The figure shows three views and two pictorial views of one solid part (mm, origin at its lowest corner). Answer the questions. A direction names the side the tool comes from. Coordinates: 2 decimals unless noted, no trailing zeros. Loops run counter-clockwise (first coordinate to the right, second up) from the corner with the lowest first, then second, coordinate; pieces in that order, holes last. Notation, with made-up numbers: (64.25, 77.5) -> (104.25, 77.5) arc R31 ccw to (104.25, 111.5) -> close; hole circle Ø1 at (-27.75, -4). An arc over 180 degrees is marked (long way). Use a Markdown table: item, result. Add a question column.
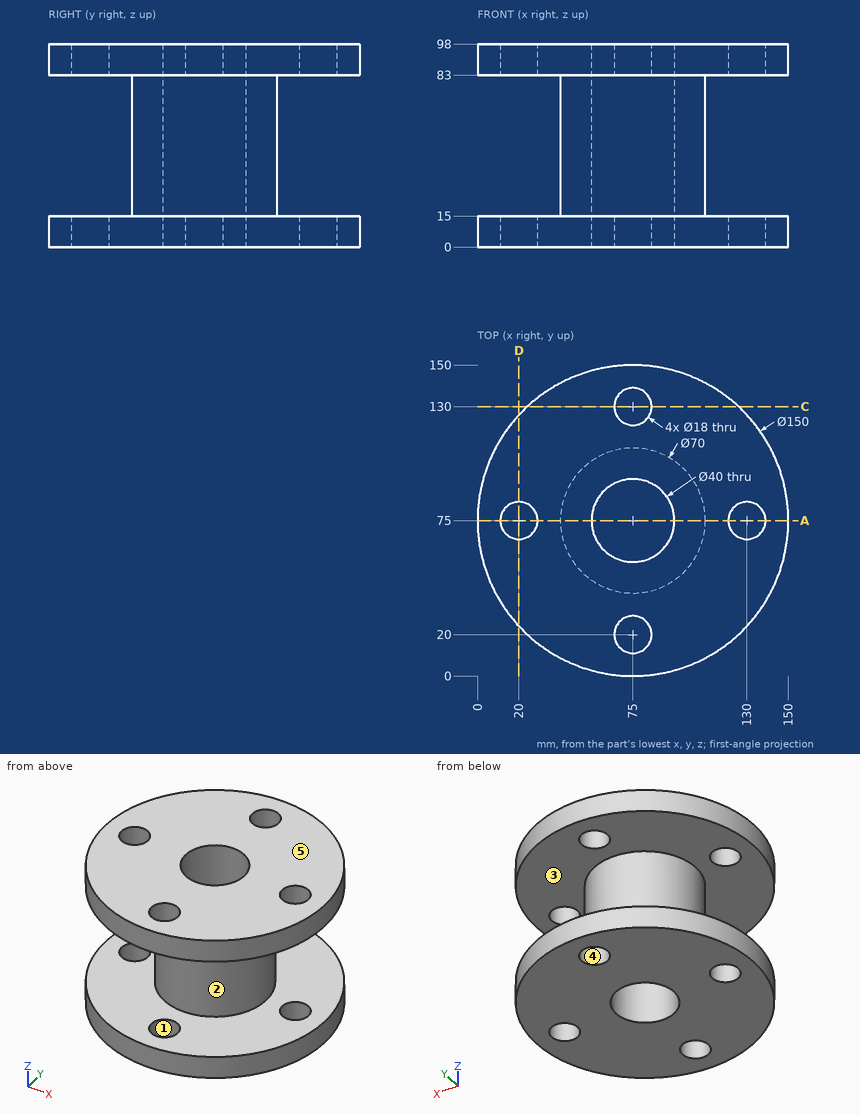
Item 1: For the marked faces 1 and 2, determine the directions among +Z, -Z, +X, -X, +Y, -Y from which every point of the face is accessible in a straight line to the end or side of a thin tool.
Item 2: Find the intervals of material crossed by probe 1 along Y at (x, z) = (75, 6.5); probe 2 along Z at (x, y) = (32.5, 57); probe 3 along Y at (x, z) = (82.5, 4), in increasing order.
Item 3: Section A-A (y = 75) is taken. Count the separate pieces of the cut face and the enclosed holes in it, then the cut area to 3 significant figures.
Item 4: For a pull along Z with two mould halves and no side action, classify the marked faces 3, 4 and 5 as +Z half, -Z half, draft (parallel to the pull), parting line (faces both ways), or undercut.
Item 5: Section C-C (y = 130) is taken. Determine the outline of the cut face in (x, z), then the cut area to 3 significant figures.
Item 6: Given pin 1 (3 mm diameter, centred on y = 79, z = 75.5, fed in from +X); pin 2 (4 mm diameter, centred on y = 89, z = 82.5, fed in from +X); pin 3 (6 mm diameter, centred on y = 56.5, z = 46.5, fed in from +X), each flat-ended and moving along its own axis, determine where each tip first touches the part or whether it passes through.
Output:
| question | item | result |
|---|---|---|
| 1 | face 1 | +Z, -Z |
| 1 | face 2 | none |
| 2 | probe 1 | y = 0 to 11, 29 to 55, 95 to 121, 139 to 150 |
| 2 | probe 2 | z = 0 to 15, 83 to 98 |
| 2 | probe 3 | y = 0.38 to 15.03, 24.97 to 56.46, 93.54 to 125.03, 134.97 to 149.62 |
| 3 | separate pieces | 6 |
| 3 | enclosed holes | 0 |
| 3 | area | 4,260 mm2 |
| 4 | face 3 | undercut |
| 4 | face 4 | draft |
| 4 | face 5 | +Z half |
| 5 | outline | (24.01, 0) -> (66, 0) -> (66, 15) -> (24.01, 15) -> close; (24.01, 83) -> (66, 83) -> (66, 98) -> (24.01, 98) -> close; (84, 0) -> (125.99, 0) -> (125.99, 15) -> (84, 15) -> close; (84, 83) -> (125.99, 83) -> (125.99, 98) -> (84, 98) -> close |
| 5 | area | 2,520 mm2 |
| 6 | pin 1 | stops at x = 109.91 |
| 6 | pin 2 | stops at x = 149.02 |
| 6 | pin 3 | stops at x = 106.38 |
